Verification items for this drawing (mm, ordinates from the low corner). Coordinates: 2 decimals unless noted, no trailing zeros. Order: outer loops, then holes, each group sorted by start corner. A loop starts at its lowest first (then second) coordinate and runs counter-clockwise, first axis right, second up. Notation, with made-up numbers: (31, 27.5) -> (73, 27.5) arc R10 ccw to (73, 39.5) -> close; hole circle Ø2 at (-38.5, -17.5). An arc over 180 degrees is marked (long way). Write each question's results on one line, items separated by ' | '. Start each with the question number.
(1) Cross-section at C-C on z = 0.7. Enter the section's corners in (x, y), and give its area (3 significant figures).
(2) Go/stop test with flat-tipped pins: pin 1 (5 mm diameter, centred on x = 32, y = 7, fed in from -Z); pin 2 (7 mm diameter, centred on x = 6.3, y = 7, fed in from +Z); pin 3 (1.2 mm diameter, centred on x = 23.5, z = 3, fed in from -Y). Record where each tip stops, or that it passes through.
(3) Cross-section at A-A on x = 32. Enter the section's corners in (y, z), and give its area (3 significant figures).
(4) Draft check along X on the marked faces 1, 2 and 3. Enter one of: +X half, -X half, draft (parallel to the pull), parting line (faces both ways), or undercut.
(5) Cross-section at B-B on y = 7. Enter the section's corners in (x, z), and give its area (3 significant figures).
(6) Thickness scan on probe 1 along Y at (x, z) = (6.3, 0.85); probe 2 along X at (y, z) = (9, 2); probe 3 along X at (y, z) = (6, 0.65). Record the ranges inside material, lowest first. Write a range as [from, to].
(7) Cross-section at D-D on y = 10.75. Enter the section's corners in (x, z), and give its area (3 significant figures).
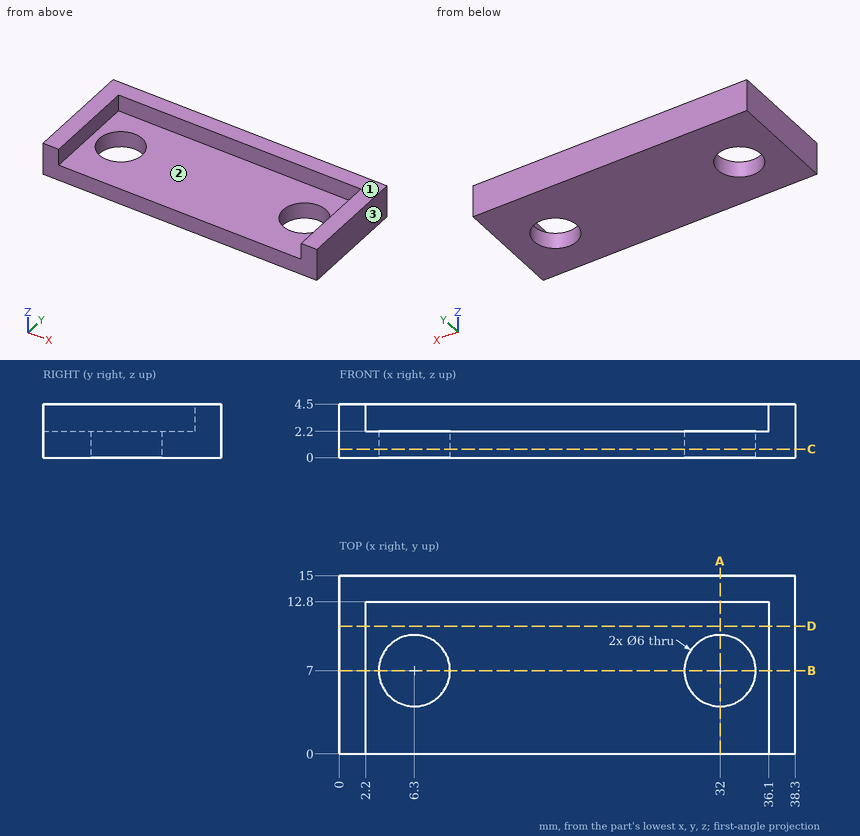
Results are:
1) outline: (0, 0) -> (38.3, 0) -> (38.3, 15) -> (0, 15) -> close; hole circle Ø6 at (6.3, 7); hole circle Ø6 at (32, 7) | area: 518 mm2
2) pin 1: passes through | pin 2: stops at z = 2.2 | pin 3: stops at y = 12.8
3) outline: (0, 0) -> (4, 0) -> (4, 2.2) -> (0, 2.2) -> close; (10, 0) -> (15, 0) -> (15, 4.5) -> (12.8, 4.5) -> (12.8, 2.2) -> (10, 2.2) -> close | area: 24.9 mm2
4) face 1: draft | face 2: undercut | face 3: +X half
5) outline: (0, 0) -> (3.3, 0) -> (3.3, 2.2) -> (2.2, 2.2) -> (2.2, 4.5) -> (0, 4.5) -> close; (9.3, 0) -> (29, 0) -> (29, 2.2) -> (9.3, 2.2) -> close; (35, 0) -> (38.3, 0) -> (38.3, 4.5) -> (36.1, 4.5) -> (36.1, 2.2) -> (35, 2.2) -> close | area: 68.0 mm2
6) probe 1: y = [0, 4], [10, 15] | probe 2: x = [0, 4.06], [8.54, 29.76], [34.24, 38.3] | probe 3: x = [0, 3.47], [9.13, 29.17], [34.83, 38.3]
7) outline: (0, 0) -> (38.3, 0) -> (38.3, 4.5) -> (36.1, 4.5) -> (36.1, 2.2) -> (2.2, 2.2) -> (2.2, 4.5) -> (0, 4.5) -> close | area: 94.4 mm2
